from build123d import *

# Parameters (mm, degrees)
SKETCH1_W               = 65.5
SKETCH1_H               = 65.5
BOSS_EXTRUDE1_DEPTH     = 3
FILLET1_R               = 3
SKETCH2_R               = 3.6
CUT_EXTRUDE1_DEPTH      = 23
SKETCH3_R               = 4.5
BOSS_EXTRUDE2_DEPTH     = 6
SKETCH4_R               = 3.6
CUT_EXTRUDE2_DEPTH      = 7
CUT_EXTRUDE2_DEPTH_BACK = 4


with BuildPart() as part:
    # Sketch1 → Boss-Extrude1 (new body)
    with BuildSketch(Plane(origin=(0, 0, 0), x_dir=(1, 0, 0), z_dir=(0, 1, 0))):
        Rectangle(SKETCH1_W, SKETCH1_H)
    extrude(amount=BOSS_EXTRUDE1_DEPTH)

    # Fillet1
    fillet1_edges = [part.edges().sort_by_distance(p)[0] for p in [
        (-32.75, 1.5, -32.75),
        (32.75, 1.5, -32.75),
        (32.75, 1.5, 32.75),
        (-32.75, 1.5, 32.75),
    ]]
    fillet(fillet1_edges, radius=FILLET1_R)

    # Sketch2 → Cut-Extrude1 (cut)
    with BuildSketch(Plane(origin=(0, 3, 0), x_dir=(1, 0, 0), z_dir=(0, 1, 0))):
        with Locations((19.85, -20)):
            Circle(SKETCH2_R)
        with Locations((19.85, 20)):
            Circle(SKETCH2_R)
    cut_extrude1 = extrude(amount=-CUT_EXTRUDE1_DEPTH, mode=Mode.SUBTRACT)

    # Mirror1: Cut-Extrude1 across plane
    add(cut_extrude1.mirror(Plane(origin=(0, 0, 0), x_dir=(0, 0, 1), z_dir=(1, 0, 0))), mode=Mode.SUBTRACT)

    # Sketch3 → Boss-Extrude2 (add)
    with BuildSketch(Plane(origin=(0, 3, 0), x_dir=(1, 0, 0), z_dir=(0, 1, 0))):
        with Locations((19.85, -20)):
            Circle(SKETCH3_R)
        with Locations((19.85, 20)):
            Circle(SKETCH3_R)
        with Locations((-19.85, 20)):
            Circle(SKETCH3_R)
        with Locations((-19.85, -20)):
            Circle(SKETCH3_R)
    extrude(amount=BOSS_EXTRUDE2_DEPTH)

    # Sketch4 → Cut-Extrude2 (cut, two sides)
    with BuildSketch(Plane(origin=(0, 3, 0), x_dir=(1, 0, 0), z_dir=(0, 1, 0))) as cut_extrude2_sk:
        with Locations((19.85, 0)):
            Circle(SKETCH4_R)
        with Locations((-19.85, 0)):
            Circle(SKETCH4_R)
    extrude(amount=CUT_EXTRUDE2_DEPTH, mode=Mode.SUBTRACT)
    extrude(cut_extrude2_sk.sketch, amount=-CUT_EXTRUDE2_DEPTH_BACK, mode=Mode.SUBTRACT)


solid = part.part
Can you work these out from the model? Positions are in its coordinate system, mm. A direction names the side the tool comes from. Coordinates: 2 decimals unless noted, no trailing zeros. Write each loop counter-clockwise with the first axis right and the second up, starting at its lowest first coordinate (ties: lowest second). Pieces come first, ordered by that corner, then holes. Notation, with made-up numbers: (18, 62) - (77, 62) arc R32 cw to (77, 92) - close; hole circle Ø4 at (33, 8.5). An arc over 180 degrees is marked (long way). Return JSON: item names as keys, results as strings. Group by question number.
Item 1: Which directions (+Z, -Z, +X, -X, +Y, -Y) give clear straight access to the entire face, cutting with the end or side of a thin tool? Please do faces 1 (the face through (-31.89, 1.52, 31.85)), 2 (the face through (0, 3, 0)), 3 (the face through (21.5, 1.5, -16.8)).
Item 2: If we section it at B-B (x = 19.85): Write out the boundary of the cut face in (y, z), then the cut area to 3 significant figures.
Item 3: Please list where these lines run through material, in increasing order: probe 1 along X at (y, z) = (2, 0); probe 2 along Z at (x, y) = (-19.85, 1.7); probe 3 along Y at (x, z) = (23, 28).
Item 4: If we section it at C-C (y = 4): Write out the boundary of the cut face in (x, z).
Item 5: I'm going to push flat-ended pins straight in: pin 1 Ø4.5 at (x, z) = (-19.85, 20) entering from -Y; pin 2 Ø9.5 at (x, z) = (-19.85, 0) entering from +Y. Where does each tip first touch, or does it pass through?
Item 6: We'd pull the mould along Z, two halves only. Please class faces 4 (the face through (20, 9, -20)), 5 (the face through (24.142, 5.958, 18.648)), 6 (the face through (31.85, 1.52, 31.89)): pulls with the +Z half, pulls with the -Z half, needs draft (parallel to the pull), parting line crosses it, or undercut.
Item 7: If we section it at D-D (z = -20): Write out the boundary of the cut face in (x, y).
Item 8: If we section it at A-A (z = 0): Write out the boundary of the cut face in (x, y).
Return value:
{
 "1": {"face 1": "+Z, -X, +Y, -Y", "face 2": "+Y", "face 3": "-Y"},
 "2": {"outline": "(0, -32.75) - (3, -32.75) - (3, -24.5) - (9, -24.5) - (9, -15.5) - (3, -15.5) - (3, -3.6) - (0, -3.6) - (0, -16.4) - (3, -16.4) - (3, -23.6) - (0, -23.6) - close; (0, 3.6) - (3, 3.6) - (3, 15.5) - (9, 15.5) - (9, 24.5) - (3, 24.5) - (3, 32.75) - (0, 32.75) - (0, 23.6) - (3, 23.6) - (3, 16.4) - (0, 16.4) - close", "area": "240 mm^2"},
 "3": {"probe 1": "x = -32.75 to -23.45, -16.25 to 16.25, 23.45 to 32.75", "probe 2": "z = -32.75 to -23.6, -16.4 to -3.6, 3.6 to 16.4, 23.6 to 32.75", "probe 3": "y = 0 to 3"},
 "4": {"outline": "circle Ø9 at (-19.85, -20); circle Ø9 at (-19.85, 20); circle Ø9 at (19.85, -20); circle Ø9 at (19.85, 20)"},
 "5": {"pin 1": "stops at y = 3", "pin 2": "stops at y = 3"},
 "6": {"face 4": "needs draft", "face 5": "undercut", "face 6": "pulls with the +Z half"},
 "7": {"outline": "(-32.75, 0) - (-23.45, 0) - (-23.45, 3) - (-16.25, 3) - (-16.25, 0) - (16.25, 0) - (16.25, 3) - (23.45, 3) - (23.45, 0) - (32.75, 0) - (32.75, 3) - (24.35, 3) - (24.35, 9) - (15.35, 9) - (15.35, 3) - (-15.35, 3) - (-15.35, 9) - (-24.35, 9) - (-24.35, 3) - (-32.75, 3) - close"},
 "8": {"outline": "(-32.75, 0) - (-23.45, 0) - (-23.45, 3) - (-32.75, 3) - close; (-16.25, 0) - (16.25, 0) - (16.25, 3) - (-16.25, 3) - close; (23.45, 0) - (32.75, 0) - (32.75, 3) - (23.45, 3) - close"}
}
